from build123d import *

# Parameters (mm, degrees)
SKETCH1_W           = 25.4
SKETCH1_H           = 152.4
BOSS_EXTRUDE1_DEPTH = 2.9718
SKETCH7_R           = 3.175
SKETCH7_W           = 6.35
SKETCH7_H           = 6.35
SKETCH7_W_2         = 3.175
CUT_EXTRUDE5_DEPTH  = 78.308224629


with BuildPart() as part:
    # Sketch1 → Boss-Extrude1 (new body)
    with BuildSketch(Plane(origin=(0, 0, 0), x_dir=(0, 1, 0), z_dir=(0, 0, 1))):
        Rectangle(SKETCH1_W, SKETCH1_H)
    extrude(amount=BOSS_EXTRUDE1_DEPTH)

    # Sketch7 → Cut-Extrude5 (cut, through all)
    with BuildSketch(Plane.XY.offset(2.9718)):
        with Locations((-50.8, 0)):
            Circle(SKETCH7_R)
        with Locations((63.5, 0)):
            Circle(SKETCH7_R)
        with Locations((-76.2, 0)):
            Rectangle(SKETCH7_W, SKETCH7_H)
        with Locations((20.6375, 0.008508047)):
            Rectangle(SKETCH7_W_2, SKETCH7_H)
    extrude(amount=-CUT_EXTRUDE5_DEPTH, mode=Mode.SUBTRACT)


solid = part.part
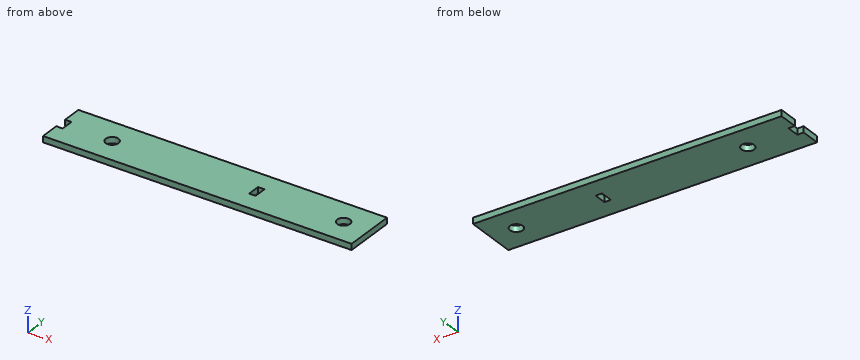
Work out the finished part from the listing and answer in its coordinate system (mm). Coordinates: 2 decimals unless noted, no trailing zeros. Write each loop counter-clockwise with the first axis right and the second up, starting at its lowest first coordinate (ties: lowest second). Pieces come first, ordered by that corner, then holes.
1. Consider line 1 along X through (y, z) = (-0.5, 1.8) (3 decimals); line 2 along Y through (x, z) = (-50.8, 2.3) (3 decimals); line 3 along X through (y, z) = (-1.5, 0.65) (3 decimals). Determine where each line is inside the solid, lowest interval first.
Results list:
line 1: x = -73.025 to -53.935, -47.665 to 19.05, 22.225 to 60.365, 66.635 to 76.2
line 2: y = -12.7 to -3.175, 3.175 to 12.7
line 3: x = -73.025 to -53.598, -48.002 to 19.05, 22.225 to 60.702, 66.298 to 76.2
2. The part is cut by section B-B, the plane y = 0. Write down the section's boundary in (x, z) (3 decimals).
Results list:
outline: (-73.025, 0) - (-53.975, 0) - (-53.975, 2.972) - (-73.025, 2.972) - close; (-47.625, 0) - (19.05, 0) - (19.05, 2.972) - (-47.625, 2.972) - close; (22.225, 0) - (60.325, 0) - (60.325, 2.972) - (22.225, 2.972) - close; (66.675, 0) - (76.2, 0) - (76.2, 2.972) - (66.675, 2.972) - close
3. The part is cut by section C-C, the plane z = 1.05. State how many separate pieces and enclosed holes the cut face has, and give its area (3 significant figures).
Results list:
separate pieces: 1
enclosed holes: 3
area: 3,770 mm2
4. The part is cut by section A-A, the plane x = -50.8. Write down the section's boundary in (y, z) (3 decimals), and give its area (3 significant figures).
Results list:
outline: (-12.7, 0) - (-3.175, 0) - (-3.175, 2.972) - (-12.7, 2.972) - close; (3.175, 0) - (12.7, 0) - (12.7, 2.972) - (3.175, 2.972) - close
area: 56.6 mm2
